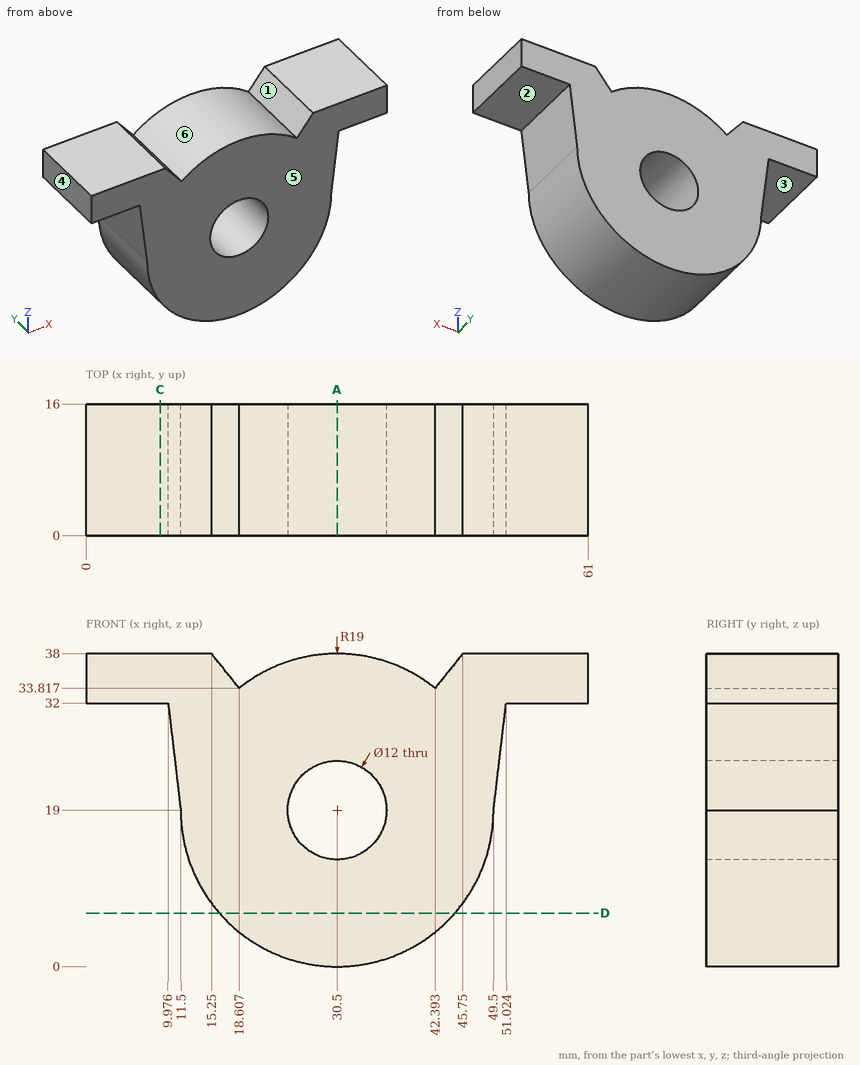
Check sheet for the drawn part. Datum: minimum x, y, z corner. Units: mm. A direction names the side the tool comes from. Round coordinates to 2 decimals unless told otherwise and drop trailing zeros. Order: outer loops, then holes, each group sorted by start corner. A loop starts at its lowest first (then second) coordinate and runs counter-clockwise, first axis right, second up.
1. Section check A-A on x = 30.5. Record the cut outline in (y, z).
Final values:
outline: (0, 0) - (16, 0) - (16, 13) - (0, 13) - close; (0, 25) - (16, 25) - (16, 38) - (0, 38) - close
2. Go/stop test with flat-tipped pins: P1, Ø6, axis at x = 19, y = 13, coming from the +Z side (1 decimal); P2, Ø6, axis at x = 38, y = 14, coming from the -Z side; P3, Ø8, axis at y = 5, z = 16, coming from the +X side. Record where each tip stops, or that it passes through.
Final values:
P1: stops at z = 37.1
P2: stops at z = 0.54
P3: stops at x = 49.62
3. Section check D-D on z = 6.5. Record the cut outline in (x, y).
Final values:
outline: (16.19, 0) - (44.81, 0) - (44.81, 16) - (16.19, 16) - close
4. Access from +Z, -Z, +X, -X, +Y, -Y to the whole of each face (thin tool, end or side, straight path). Record for the marked faces 1, 2 and 3.
Final values:
face 1: +Z, +Y, -Y
face 2: -Z, +X, +Y, -Y
face 3: -Z, -X, +Y, -Y
5. Release check for a two-part mould opening along X. For the marked faces 4, 5 and 6 record: +X half, -X half, draft (parallel to the pull), parting line (faces both ways), or undercut.
Final values:
face 4: -X half
face 5: draft
face 6: undercut
6. Section check C-C on x = 9. Record the cut outline in (y, z).
Final values:
outline: (0, 32) - (16, 32) - (16, 38) - (0, 38) - close
7. Thickness scan on L1, parallel to X at y = 3.5, z = 19; L2, parallel to X at y = 1.25, z = 23; L3, parallel to X at y = 13, z = 34.5 (1 decimal). Record the ranges inside material, lowest first.
Final values:
L1: x = 11.5 to 24.5, 36.5 to 49.5
L2: x = 11.03 to 26.03, 34.97 to 49.97
L3: x = 0 to 18.1, 19.5 to 41.5, 42.9 to 61
